Design review of the part built by this model. Coordinates are the model's own, in mm. A direction names the side the tool comes from. Coordinates: 2 decimals unless noted, no trailing zeros. Loops run counter-clockwise (first coordinate to the right, second up) from the corner with the lowest first, then second, coordinate; pieces in that order, holes last. Notation, with made-up numbers: M 34.5,0.5 L 56.5,0.5 A27 cw 56.5,27.5 Z; hole C 5,48.25 d8. An arc over 180 degrees is marked long. Write item = value, one per line. Start each with the question number.
from build123d import *

# Parameters (mm, degrees)
EXTRUDE_START   = -2
EXTRUDE_1_DEPTH = 32
SHELL_1_T       = -2
FILLET_1_R      = 5


with BuildPart() as part:
    # 草图1 → 凸台-拉伸1 (new body)
    with BuildSketch(Plane(origin=(0, 0, 0), x_dir=(1, 0, 0), z_dir=(0, 1, 0)).offset(EXTRUDE_START)):
        with BuildLine():
            Line((-97.488460856, 50), (-69, 50))
            ThreePointArc((-69, 50), (-65, 46), (-61, 50))
            Line((-61, 50), (-7.5, 50))
            Line((-7.5, 50), (7.5, 50))
            Line((7.5, 50), (61, 50))
            ThreePointArc((61, 50), (65, 46), (69, 50))
            Line((69, 50), (97.488460856, 50))
            ThreePointArc((97.488460856, 50), (70.958011296, -7.594087263), (14.719298061, -36.888297872))
            ThreePointArc((14.719298061, -36.888297872), (0, -49), (-14.719298061, -36.888297872))
            ThreePointArc((-14.719298061, -36.888297872), (-70.958011296, -7.594087263), (-97.488460856, 50))
        make_face()
    extrude(amount=EXTRUDE_1_DEPTH)

    # 抽壳1
    shell_1_openings = [part.faces().sort_by_distance(p)[0] for p in [
        (0, 30, -11.801216643),
    ]]
    offset(amount=SHELL_1_T, openings=shell_1_openings, kind=Kind.INTERSECTION)

    # 圆角1
    fillet_1_edges = [part.edges().sort_by_distance(p)[0] for p in [
        (14.719298061, 14, 36.888297872),
        (-14.719298061, 14, 36.888297872),
        (-12.951461384, 15, 35.122340426),
        (12.951461384, 15, 35.122340426),
    ]]
    fillet(fillet_1_edges, radius=FILLET_1_R)


solid = part.part
Q1. To check wall thickness, follow line 1 (Z direction, x = 1, y = 2); line 2 (Z direction, x = -88.5, y = 23); line 3 (X direction, y = 1, z = 10.5). State the ranges of each line that lie inside material, in increasing order. Write a range as from..to.
Q2. For faces 5 (the face through (1, -2, -12)), 6 (the face through (-68.8, 14.79, 6.95)), list the 3-axis set-ups (+Z, -Z, +X, -X, +Y, -Y) from which the entire face can be reached by the end or side of a thin tool; tool diameter is ignored.
Q3. Add section A-A on z = 8.5. State the section outline as (x, y) points.
Q4. Clearance check with flat-ended pins moving along their axes: P1, Ø12, axis at x = -66.5, y = 6, coming from the +Z side; P2, Ø8, axis at y = 4, z = 7, coming from the -X side; P3, Ø12.5, axis at x = 85.5, y = 22, coming from the +Z side. State where each tip first meets the part, or that it passes through.
Q5. Add section B-B on x = 44.5. State the section outline as (y, z) points, plus the area to 3 significant figures.
Q6. Mouldability with a two-part tool opening along Z and no side actions: class faces 1 (the face through (7.7, 30, -48.4)), 2 (the face through (-65, 14, -46)), 3 (the face through (72.59, 13.78, 5.84)), 4 (the face through (1, 0, -12)) as released by +Z, released by -Z, zero draft, split by the parting line, or undercut.
Values follow:
q1.line_1 = -50..-48, 46.96..48.97
q1.line_2 = -50..-48, -22.8..-17.91
q1.line_3 = -68.07..-65.16, 65.16..68.07
q2.face_5 = +Z, -Z, +X, -X, -Y
q2.face_6 = +Y
q3.outline = M -70.08,-2 L 70.08,-2 L 70.08,30 L 67.26,30 L 67.26,0 L -67.26,0 L -67.26,30 L -70.08,30 Z
q4.P1 = 17.1
q4.P2 = -75.07
q4.P3 = -2.35
q5.outline = M -2,-50 L 30,-50 L 30,-48 L 0,-48 L 0,25.06 L 30,25.06 L 30,27.31 L -2,27.31 Z
q5.area = 282 mm2
q6.face_1 = zero draft
q6.face_2 = released by -Z
q6.face_3 = released by +Z
q6.face_4 = undercut
